```python
from build123d import *

# Parameters (mm, degrees)
SKETCH_W        = 62.5
SKETCH_H        = 36.5
PAD_DEPTH       = 9
SKETCH001_W     = 58.5
SKETCH001_H     = 32.5
POCKET_DEPTH    = 7
SKETCH002_R     = 3.09059
PAD001_DEPTH    = 6.5
SKETCH003_R     = 1.8
POCKET001_DEPTH = 3.5
SKETCH004_W     = 4
SKETCH004_H     = 2.125
POCKET002_DEPTH = 3
SKETCH005_W     = 9.2
SKETCH005_H     = 4.7
POCKET003_DEPTH = 5
FILLET_R        = 1.2
FILLET001_R     = 1.2
POCKET004_DEPTH = 5
SKETCH007_W     = 30.5
SKETCH007_H     = 0.6
POCKET005_DEPTH = 2
SKETCH008_W     = 58.5
SKETCH008_H     = 0.6
POCKET006_DEPTH = 2
SKETCH009_W     = 24
SKETCH009_H     = 0.6
POCKET007_DEPTH = 2
SKETCH010_W     = 0.6
SKETCH010_H     = 3
POCKET008_DEPTH = 2
SKETCH011_W     = 0.6
SKETCH011_H     = 3
POCKET009_DEPTH = 2
FILLET002_R     = 2
FILLET003_R     = 1


with BuildPart() as part:
    # Sketch → Pad (new body)
    with BuildSketch(Plane.XY):
        Rectangle(SKETCH_W, SKETCH_H)
    extrude(amount=PAD_DEPTH)

    # Sketch001 (on Face5 of Pad) → Pocket (cut)
    with BuildSketch(Plane(origin=(0, 0, 0), x_dir=(1, 0, 0), z_dir=(0, 0, -1))):
        Rectangle(SKETCH001_W, SKETCH001_H)
    extrude(amount=-POCKET_DEPTH, mode=Mode.SUBTRACT)

    # Sketch002 (on Face11 of Pocket) → Pad001 (join)
    with BuildSketch(Plane(origin=(0, 0, 7), x_dir=(1, 0, 0), z_dir=(0, 0, -1))):
        with Locations((-4.037531, 0)):
            Circle(SKETCH002_R)
    extrude(amount=PAD001_DEPTH)

    # Sketch003 (on Face13 of Pad001) → Pocket001 (cut)
    with BuildSketch(Plane(origin=(0, 0, 0.5), x_dir=(1, 0, 0), z_dir=(0, 0, -1))):
        with Locations((-4.053153, 0)):
            Circle(SKETCH003_R)
    extrude(amount=-POCKET001_DEPTH, mode=Mode.SUBTRACT)

    # Sketch004 (on Face4 of Pocket001) → Pocket002 (cut)
    with BuildSketch(Plane(origin=(0, 0, 0), x_dir=(1, 0, 0), z_dir=(0, 0, -1))):
        with Locations((3.25, 17.240923)):
            Rectangle(SKETCH004_W, SKETCH004_H)
    extrude(amount=-POCKET002_DEPTH, mode=Mode.SUBTRACT)

    # Sketch005 (on Face1 of Pocket002) → Pocket003 (cut)
    with BuildSketch(Plane(origin=(-31.25, 0, 0), x_dir=(0, -1, 0), z_dir=(-1, 0, 0))):
        with Locations((0, 2.35)):
            Rectangle(SKETCH005_W, SKETCH005_H)
    extrude(amount=-POCKET003_DEPTH, mode=Mode.SUBTRACT)

    # Fillet
    fillet_edges = [part.edges().sort_by_distance(p)[0] for p in [
        (-30.25, -4.6, 4.7),
    ]]
    fillet(fillet_edges, radius=FILLET_R)

    # Fillet001
    fillet001_edges = [part.edges().sort_by_distance(p)[0] for p in [
        (-30.25, 4.6, 4.7),
    ]]
    fillet(fillet001_edges, radius=FILLET001_R)

    # Sketch006 (on Face13 of Fillet001) → Pocket004 (cut)
    with BuildSketch(Plane.YZ.offset(31.25)):
        with BuildLine():
            ThreePointArc((3.1, 3.258545), (0.041455, 6.4), (-3.1, 3.341455))
            Line((-3.1, 3.341455), (-3.1, 0))
            Line((-3.1, 0), (3.1, 0))
            Line((3.1, 3.258545), (3.1, 0))
        make_face()
        with BuildLine():
            ThreePointArc((-7.7, 3.041637), (-10.800001, 6.410748), (-13.9, 3.041636))
            Line((-13.9, 3.041636), (-13.9, 0))
            Line((-7.7, 0), (-13.9, 0))
            Line((-7.7, 3.041637), (-7.7, 0))
        make_face()
        with BuildLine():
            ThreePointArc((13.9, 3.012545), (10.799999, 6.413299), (7.7, 3.012544))
            Line((7.7, 3.012544), (7.7, 0))
            Line((13.9, 0), (7.7, 0))
            Line((13.9, 3.012545), (13.9, 0))
        make_face()
    extrude(amount=-POCKET004_DEPTH, mode=Mode.SUBTRACT)

    # Sketch007 (on Face8 of Pocket004) → Pocket005 (cut)
    with BuildSketch(Plane(origin=(0, 0, 0), x_dir=(1, 0, 0), z_dir=(0, 0, -1))):
        with Locations((-14, 16.55)):
            Rectangle(SKETCH007_W, SKETCH007_H)
    extrude(amount=-POCKET005_DEPTH, mode=Mode.SUBTRACT)

    # Sketch008 (on Face7 of Pocket004) → Pocket006 (cut)
    with BuildSketch(Plane(origin=(0, 0, 0), x_dir=(1, 0, 0), z_dir=(0, 0, -1))):
        with Locations((0, -16.55)):
            Rectangle(SKETCH008_W, SKETCH008_H)
    extrude(amount=-POCKET006_DEPTH, mode=Mode.SUBTRACT)

    # Sketch009 (on Face19 of Pocket004) → Pocket007 (cut)
    with BuildSketch(Plane(origin=(0, 0, 0), x_dir=(1, 0, 0), z_dir=(0, 0, -1))):
        with Locations((17.25, 16.55)):
            Rectangle(SKETCH009_W, SKETCH009_H)
    extrude(amount=-POCKET007_DEPTH, mode=Mode.SUBTRACT)

    # Sketch010 (on Face22 of Pocket007) → Pocket008 (cut)
    with BuildSketch(Plane(origin=(0, 0, 0), x_dir=(1, 0, 0), z_dir=(0, 0, -1))):
        with Locations((29.55, 15.35)):
            Rectangle(SKETCH010_W, SKETCH010_H)
    extrude(amount=-POCKET008_DEPTH, mode=Mode.SUBTRACT)

    # Sketch011 (on Face7 of Pocket008) → Pocket009 (cut)
    with BuildSketch(Plane(origin=(0, 0, 0), x_dir=(1, 0, 0), z_dir=(0, 0, -1))):
        with Locations((29.55, -15.35)):
            Rectangle(SKETCH011_W, SKETCH011_H)
    extrude(amount=-POCKET009_DEPTH, mode=Mode.SUBTRACT)

    # Fillet002
    fillet002_edges = [part.edges().sort_by_distance(p)[0] for p in [
        (-7.128121, 0, 7),
    ]]
    fillet(fillet002_edges, radius=FILLET002_R)

    # Fillet003
    fillet003_edges = [part.edges().sort_by_distance(p)[0] for p in [
        (31.25, -18.25, 4.5),
        (0, -18.25, 9),
        (31.25, 0, 9),
        (31.25, 18.25, 4.5),
        (0, 18.25, 9),
        (-31.25, 18.25, 4.5),
        (-31.25, 0, 9),
        (-31.25, -18.25, 4.5),
    ]]
    fillet(fillet003_edges, radius=FILLET003_R)


solid = part.part
```
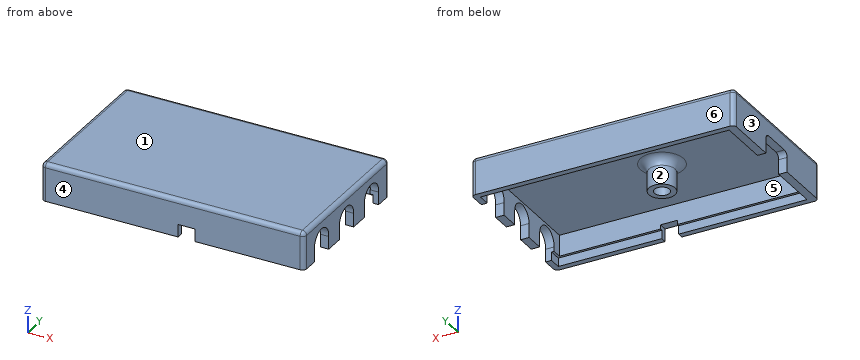
For this review, take the finished solid that the model builds, in its own axes (mm). Face numbers are marked on the shaded views. A direction names the side the tool comes from. Coordinates: 2 decimals unless noted, no trailing zeros. Write each loop counter-clockwise with the first axis right and the second up, starting at its lowest first coordinate (ties: lowest second). Pieces come first, ordered by that corner, then holes. Notation, with made-up numbers: (25, 84.25) - (53, 84.25) arc R16 cw to (53, 101.25) - close; hole circle Ø8 at (16.5, 4). An arc over 180 degrees is marked (long way). Put each result on its own line as item: value.
1. Mouldability with a two-part tool opening along Y and no side actions: class the marked faces 3, 4, 5 and 6 as released by +Y, released by -Y, zero draft, split by the parting line, or undercut.
Values found:
face 3: zero draft
face 4: released by -Y
face 5: undercut
face 6: released by +Y
2. Wall thickness on probe 1 along Y at (x, z) = (-4, 5.25); probe 2 along Y at (x, z) = (29.8, 3.3); probe 3 along X at (y, z) = (-7.5, 6.75): over which ranges is each line inside the solid? List them lowest first.
Values found:
probe 1: -18.25 to -16.25, -3.11 to 3.11, 16.25 to 18.25
probe 2: -18.25 to -13.91, -7.69 to -3.1, 3.1 to 7.69, 13.91 to 18.25
probe 3: -31.25 to -29.25, 29.25 to 31.25
3. Add section D-D, the plane y = 10.8. Give the boundary of the cut face in (x, z), then the cut area to 3 significant figures.
Values found:
outline: (-31.25, 0) - (-29.25, 0) - (-29.25, 7) - (29.25, 7) - (29.25, 6.41) - (31.25, 6.41) - (31.25, 8) arc R1 ccw to (30.25, 9) - (-30.25, 9) arc R1 ccw to (-31.25, 8) - close
area: 140 mm²
4. Machinability: for the marked faces 1 and 2, which of the approach directions +Z, -Z, +X, -X, +Y, -Y give a long, thin tool a straight path to every point of the face, cutting with its end or side? Answer none if there is none.
Values found:
face 1: +Z, +X, -X, +Y, -Y
face 2: -Z
5. Add section B-B, the plane x = -22.5. Give the boundary of the cut face in (y, z).
Values found:
outline: (-18.25, 0) - (-16.85, 0) - (-16.85, 2) - (-16.25, 2) - (-16.25, 7) - (16.25, 7) - (16.25, 2) - (16.85, 2) - (16.85, 0) - (18.25, 0) - (18.25, 8) arc R1 ccw to (17.25, 9) - (-17.25, 9) arc R1 ccw to (-18.25, 8) - close
6. For pin 1 (2 mm diameter, centred on y = -13.5, z = 3, fed in from +X); pin 2 (3.5 mm diameter, centred on y = 10.8, z = 3.3, fed in from +X); pin 3 (1.5 mm diameter, centred on x = 18.5, y = -15, fed in from -Z), all flat-tipped, find the tip position at first contact; note any pin that passes through.
Values found:
pin 1: x = 31.25
pin 2: x = -29.25
pin 3: z = 7
7. Add section C-C, the plane y = -6. Give the boundary of the cut face in (x, z), then the cut area to 3 significant figures.
Values found:
outline: (-31.25, 0) - (-29.25, 0) - (-29.25, 7) - (29.25, 7) - (29.25, 0) - (31.25, 0) - (31.25, 8) arc R1 ccw to (30.25, 9) - (-30.25, 9) arc R1 ccw to (-31.25, 8) - close
area: 153 mm²
8. Add section A-A, the plane y = 0. Give the boundary of the cut face in (x, z), then the cut area to 3 significant figures.
Values found:
outline: (-31.25, 4.7) - (-29.25, 4.7) - (-29.25, 7) - (-9.13, 7) arc R2 cw to (-7.13, 5) - (-7.13, 0.5) - (-5.85, 0.5) - (-5.85, 4) - (-2.25, 4) - (-2.25, 0.5) - (-0.95, 0.5) - (-0.95, 5) arc R2 cw to (1.05, 7) - (29.25, 7) - (29.25, 6.4) - (31.25, 6.4) - (31.25, 8) arc R1 ccw to (30.25, 9) - (-30.25, 9) arc R1 ccw to (-31.25, 8) - close
area: 160 mm²
